from build123d import *

# Parameters (mm, degrees)
SKETCH_1_W      = 40
SKETCH_1_H      = 30
SKETCH_1_R      = 1
EXTRUDE_1_DEPTH = 1.5
SKETCH_2_W      = 5
SKETCH_2_H      = 7.8
EXTRUDE_2_DEPTH = 2.5
SKETCH_3_W      = 15.5
SKETCH_3_H      = 15.5
EXTRUDE_3_DEPTH = 5
SKETCH_4_W      = 5
SKETCH_4_H      = 18
EXTRUDE_4_DEPTH = 10


with BuildPart() as part:
    # 草图1 → 凸台-拉伸1 (new body)
    with BuildSketch(Plane(origin=(0, 0, 0), x_dir=(1, 0, 0), z_dir=(0, 1, 0))):
        Rectangle(SKETCH_1_W, SKETCH_1_H)
        with Locations(Location((-17, 12, 0), (0, 0, 270))):
            Circle(SKETCH_1_R, mode=Mode.SUBTRACT)
        with Locations(Location((17, 12, 0), (0, 0, 90))):
            Circle(SKETCH_1_R, mode=Mode.SUBTRACT)
        with Locations(Location((17, -12, 0), (0, 0, 270))):
            Circle(SKETCH_1_R, mode=Mode.SUBTRACT)
        with Locations(Location((-17, -12, 0), (0, 0, 90))):
            Circle(SKETCH_1_R, mode=Mode.SUBTRACT)
    extrude(amount=EXTRUDE_1_DEPTH)

    # 草图2 → 凸台-拉伸2 (add)
    with BuildSketch(Plane(origin=(0, 1.5, 0), x_dir=(1, 0, 0), z_dir=(0, 1, 0))):
        with Locations((-17.5, 0)):
            Rectangle(SKETCH_2_W, SKETCH_2_H)
    extrude(amount=EXTRUDE_2_DEPTH)

    # 草图3 → 凸台-拉伸3 (add)
    with BuildSketch(Plane(origin=(0, 1.5, 0), x_dir=(1, 0, 0), z_dir=(0, 1, 0))):
        with Locations((-0.25, 1.75)):
            Rectangle(SKETCH_3_W, SKETCH_3_H)
    extrude(amount=EXTRUDE_3_DEPTH)

    # 草图4 → 凸台-拉伸4 (add)
    with BuildSketch(Plane(origin=(0, 1.5, 0), x_dir=(1, 0, 0), z_dir=(0, 1, 0))):
        with Locations((14.5, 0)):
            Rectangle(SKETCH_4_W, SKETCH_4_H)
    extrude(amount=EXTRUDE_4_DEPTH)


solid = part.part
Check sheet for the modelled part. Datum: model origin and axes. Units: mm. A direction names the side the tool comes from. Coordinates: 2 decimals unless noted, no trailing zeros. Loops run counter-clockwise (first coordinate to the right, second up) from the corner with the lowest first, then second, coordinate; pieces in that order, holes last. Notation, with made-up numbers: (82, 80.25) -> (93, 80.25) arc R22 ccw to (93, 119.25) -> close; hole circle Ø9 at (30.25, -12.75). An arc over 180 degrees is marked (long way). Answer in a Markdown table with one row per item.
1. Sectioned sample at A-A, the plane y = 6. Record the boundary of the cut face in (x, z), then the cut area to 3 significant figures.
Check values:
| item | result |
|---|---|
| outline | (-8, -9.5) -> (7.5, -9.5) -> (7.5, 6) -> (-8, 6) -> close; (12, -9) -> (17, -9) -> (17, 9) -> (12, 9) -> close |
| area | 330 mm2 |
2. Material ranges on line 1 along X through (y, z) = (0.85, -12); line 2 along Z through (x, y) = (-3, 3.75); line 3 along Y through (x, z) = (-9.5, -8.5), recorded low to high. Write a range as [from, to].
Check values:
| item | result |
|---|---|
| line 1 | x = [-20, -18], [-16, 16], [18, 20] |
| line 2 | z = [-9.5, 6] |
| line 3 | y = [0, 1.5] |
3. Sectioned sample at C-C, the plane x = 15.5. Record the boundary of the cut face in (y, z), then the cut area to 3 significant figures.
Check values:
| item | result |
|---|---|
| outline | (0, -15) -> (1.5, -15) -> (1.5, -9) -> (11.5, -9) -> (11.5, 9) -> (1.5, 9) -> (1.5, 15) -> (0, 15) -> close |
| area | 225 mm2 |
4. Access from +Z, -Z, +X, -X, +Y, -Y to the whole of each face (thin tool, end or side, straight path). Record for faces 5 (the face through (-18, 3, -3.9)), 6 (the face through (14, 6, -9)), 7 (the face through (-8, 4, -2)), 8 (the face through (-18, 4, 0)).
Check values:
| item | result |
|---|---|
| face 5 | -Z, -X, +Y |
| face 6 | -Z, +X, +Y |
| face 7 | +Z, -Z, +Y |
| face 8 | +Z, -Z, -X, +Y |
5. Release check for a two-part mould opening along Z. For faces 1 (the face through (-18, 3, 3.9)), 2 (the face through (18, 1, -12)), 3 (the face through (17, 6, 0)), 4 (the face through (16, 1, 12)) record: released by +Z, released by -Z, zero draft, split by the parting line, or undercut.
Check values:
| item | result |
|---|---|
| face 1 | released by +Z |
| face 2 | undercut |
| face 3 | zero draft |
| face 4 | undercut |
6. Sectioned sample at D-D, the plane z = -8.25. Record the boundary of the cut face in (x, y).
Check values:
| item | result |
|---|---|
| outline | (-20, 0) -> (20, 0) -> (20, 1.5) -> (17, 1.5) -> (17, 11.5) -> (12, 11.5) -> (12, 1.5) -> (7.5, 1.5) -> (7.5, 6.5) -> (-8, 6.5) -> (-8, 1.5) -> (-20, 1.5) -> close |
7. Sectioned sample at B-B, the plane z = 12. Record the boundary of the cut face in (x, y), then the cut area to 3 significant figures.
Check values:
| item | result |
|---|---|
| outline | (-20, 0) -> (-18, 0) -> (-18, 1.5) -> (-20, 1.5) -> close; (-16, 0) -> (16, 0) -> (16, 1.5) -> (-16, 1.5) -> close; (18, 0) -> (20, 0) -> (20, 1.5) -> (18, 1.5) -> close |
| area | 54.0 mm2 |
8. Go/stop test with flat-tipped pins: pin 1 (4 mm diameter, centred on y = 4, z = -4.5, fed in from +X); pin 2 (5.5 mm diameter, centred on x = -2.5, y = 4.5, fed in from -Z); pin 3 (5 mm diameter, centred on y = 7.5, z = 4.5, fed in from -X); pin 4 (1.8 mm diameter, centred on x = 17, z = 12, fed in from -Y). Record where each tip stops, or that it passes through.
Check values:
| item | result |
|---|---|
| pin 1 | stops at x = 17 |
| pin 2 | stops at z = -9.5 |
| pin 3 | stops at x = -8 |
| pin 4 | passes through |
